```python
from build123d import *

# Parameters (mm, degrees)
SKETCH1_W                 = 38.1
SKETCH1_H                 = 50.8
SKETCH1_W_2               = 50.8
SKETCH1_H_2               = 44.45
SKETCH1_W_3               = 6.365635467
BOSS_EXTRUDE1_DEPTH       = 3.175
TAP_DRILL_FOR_8_32_TAP1_D = 3.4544
F_4_0_4_DIAMETER_HOLE1_D  = 4
TAP_DRILL_FOR_4_40_TAP1_D = 2.2606
TAP_DRILL_FOR_4_40_TAP2_D = 2.2606


with BuildPart() as part:
    # Sketch1 → Boss-Extrude1 (new body)
    with BuildSketch(Plane(origin=(0, 0, 0), x_dir=(1, 0, 0), z_dir=(0, 1, 0))):
        with Locations((-12.7, -6.35)):
            Rectangle(SKETCH1_W, SKETCH1_H)
        with Locations((31.75, -6.35)):
            Rectangle(SKETCH1_W_2, SKETCH1_H)
        with Locations((31.75, 41.275)):
            Rectangle(SKETCH1_W_2, SKETCH1_H_2)
        with Locations((76.2, -6.35)):
            Rectangle(SKETCH1_W, SKETCH1_H)
        with Locations((98.432817734, -6.35)):
            Rectangle(SKETCH1_W_3, SKETCH1_H)
    extrude(amount=BOSS_EXTRUDE1_DEPTH)

    # Tap Drill for #8-32 Tap1 (through all)
    with Locations(Plane(origin=(-12.7, 3.175, 0), x_dir=(0, 0, 1), z_dir=(0, 1, 0))):
        with Locations((0, 0), (0, -12.7), (12.7, -12.7), (25.4, -12.7), (25.4, 0), (-12.7, 0), (-12.7, -12.7), (12.7, 0)):
            Hole(TAP_DRILL_FOR_8_32_TAP1_D / 2)

    # Ø4.0 (4) Diameter Hole1 (through all)
    with Locations(Plane(origin=(31.75, 3.175, -12.15), x_dir=(0, 0, 1), z_dir=(0, 1, 0))):
        with Locations((0, 0), (9.25, 16.02146997), (27.75, 16.02146997), (37, 0), (27.75, -16.02146997), (9.25, -16.02146997)):
            Hole(F_4_0_4_DIAMETER_HOLE1_D / 2)

    # Tap Drill for #4-40 Tap1 (through all)
    with Locations(Plane(origin=(69.865635467, 3.175, -6.35), x_dir=(0, 0, 1), z_dir=(0, 1, 0))):
        with Locations((0, 0), (0, 25.4), (25.4, 25.4), (25.4, 0)):
            Hole(TAP_DRILL_FOR_4_40_TAP1_D / 2)

    # Tap Drill for #4-40 Tap2 (through all)
    with Locations(Plane(origin=(31.75, 3.175, -53.975), x_dir=(0, 0, 1), z_dir=(0, 1, 0))):
        with Locations((0, 0), (25.4, 0)):
            Hole(TAP_DRILL_FOR_4_40_TAP2_D / 2)


solid = part.part
```
Read the model definition and answer for the solid it produces. Units are mm, in the model's axes. A direction names the side the tool comes from. Coordinates: 2 decimals unless noted, no trailing zeros. Write each loop counter-clockwise with the first axis right and the second up, starting at its lowest first coordinate (ties: lowest second). Pieces come first, ordered by that corner, then holes. Notation, with made-up numbers: (45, 9) - (49, 9) arc R27 cw to (49, 40) - close; hole circle Ø5 at (-32.5, 41.25). An arc over 180 degrees is marked (long way). Answer as a JSON object with one key per item and string values. Group by question number.
1. Which of the six approach directions +Z, -Z, +X, -X, +Y, -Y give full straight-line access (tool end or side, diameter ignored) to faces 5 (the cylindrical face through (29.976, 1.565, 23.927)), 6 (the flat face through (6.35, 2, -41)), 7 (the flat face through (57.15, 2, -41))?
2. A cutting plane is placed at D-D (x = 66.5). Determine the outline of the cut face in (y, z) (3 decimals).
3. Consider L1, parallel to X at y = 2.15, z = -2.9; L2, parallel to X at y = 1.7, z = 25.4; L3, parallel to Z at x = 94.5, y = 2.05. Determine where each line is inside the solid, lowest interval first. Write a range as [from, to].
4. A cutting plane is placed at C-C (y = 1.35). Give the number of separate pieces and of enclosed holes in the cut face, plus the area to 3 significant figures.
5. A cutting plane is placed at B-B (z = -12.7). Determine the outline of the cut face in (x, y) (3 decimals), plus the area to 3 significant figures.
6. The mould has two halves that part along X. Classify faces 1 (the flat face through (-31.75, 2, 7)), 2 (the flat face through (-12, 2, -19.05)), 3 (the cylindrical face through (-12.181, 1.565, -14.347)), 4 (the cylindrical face through (-23.687, 1.565, 0.225)): +X half, -X half, draft (parallel to the pull), parting line (faces both ways), or undercut.
7. Each of these flat-tipped pins is pushed along its axis until it touches: P1, Ø1.5, axis at x = -1.5, y = 1, coming from the -Z side; P2, Ø1.6, axis at y = 1.5, z = -44.5, coming from the +X side; P3, Ø1, axis at x = 79.5, z = 0.5, coming from the -Y side. Where does it stop, or does it pass through?
8. A cutting plane is placed at A-A (x = -12.7). Determine the outline of the cut face in (y, z) (3 decimals).
Worked out:
{
 "1": {"face 5": "+Y, -Y", "face 6": "-Z, -X, +Y, -Y", "face 7": "-Z, +X, +Y, -Y"},
 "2": {"outline": "(0, -19.05) - (3.175, -19.05) - (3.175, 31.75) - (0, 31.75) - close"},
 "3": {"L1": "x = [-31.75, 13.73], [17.73, 45.77], [49.77, 101.62]", "L2": "x = [-31.75, -27.13], [-23.67, -14.43], [-10.97, 29.83], [33.67, 101.62]", "L3": "z = [-19.05, -7.18], [-5.52, 18.22], [19.88, 31.75]"},
 "4": {"separate pieces": "1", "enclosed holes": "20", "area": "8,860 mm²"},
 "5": {"outline": "(-31.75, 0) - (-27.127, 0) - (-27.127, 3.175) - (-31.75, 3.175) - close; (-23.673, 0) - (-14.427, 0) - (-14.427, 3.175) - (-23.673, 3.175) - close; (-10.973, 0) - (29.827, 0) - (29.827, 3.175) - (-10.973, 3.175) - close; (33.673, 0) - (101.616, 0) - (101.616, 3.175) - (33.673, 3.175) - close", "area": "389 mm²"},
 "6": {"face 1": "-X half", "face 2": "draft", "face 3": "undercut", "face 4": "undercut"},
 "7": {"P1": "stops at z = -19.05", "P2": "stops at x = 57.15", "P3": "stops at y = 0"},
 "8": {"outline": "(0, -19.05) - (3.175, -19.05) - (3.175, -14.427) - (0, -14.427) - close; (0, -10.973) - (3.175, -10.973) - (3.175, -1.727) - (0, -1.727) - close; (0, 1.727) - (3.175, 1.727) - (3.175, 10.973) - (0, 10.973) - close; (0, 14.427) - (3.175, 14.427) - (3.175, 23.673) - (0, 23.673) - close; (0, 27.127) - (3.175, 27.127) - (3.175, 31.75) - (0, 31.75) - close"}
}
